from build123d import *

# Parameters (mm, degrees)
F1_DEPTH = 12
F2_SIZE  = 10


with BuildPart() as f1:
    # F0 (on Front) → F1 (new body)
    with BuildSketch(Plane.XZ):
        with BuildLine():
            Line((1, -45), (45, -45))
            Line((45, -45), (45, 45))
            Line((45, 45), (1, 45))
            Line((1, 45), (1, 24.096539))
            ThreePointArc((1, 24.096539), (0, 23.096539), (-1, 24.096539))
            Line((-1, 24.096539), (-1, 45))
            Line((-1, 45), (-45, 45))
            Line((-45, 45), (-45, -45))
            Line((-45, -45), (-1, -45))
            Line((-1, -45), (-1, -24.096539))
            ThreePointArc((-1, -24.096539), (0, -23.096539), (1, -24.096539))
            Line((1, -24.096539), (1, -45))
        make_face()
        with BuildLine():
            ThreePointArc((-6.732051, -7.660254), (-4, -6.928203), (-3.267949, -9.660254))
            Line((-3.267949, -9.660254), (-15.767949, -31.310889))
            ThreePointArc((-15.767949, -31.310889), (-18.5, -32.04294), (-19.232051, -29.310889))
            Line((-19.232051, -29.310889), (-6.732051, -7.660254))
        make_face(mode=Mode.SUBTRACT)
        with BuildLine():
            ThreePointArc((3.267949, -9.660254), (4, -6.928203), (6.732051, -7.660254))
            Line((6.732051, -7.660254), (19.232051, -29.310889))
            ThreePointArc((19.232051, -29.310889), (18.5, -32.04294), (15.767949, -31.310889))
            Line((15.767949, -31.310889), (3.267949, -9.660254))
        make_face(mode=Mode.SUBTRACT)
        with BuildLine():
            Line((-35, 2), (-10, 2))
            ThreePointArc((-10, 2), (-8, 0), (-10, -2))
            Line((-10, -2), (-35, -2))
            ThreePointArc((-35, -2), (-37, 0), (-35, 2))
        make_face(mode=Mode.SUBTRACT)
        with BuildLine():
            ThreePointArc((-3.267949, 9.660254), (-4, 6.928203), (-6.732051, 7.660254))
            Line((-6.732051, 7.660254), (-19.232051, 29.310889))
            ThreePointArc((-19.232051, 29.310889), (-18.5, 32.04294), (-15.767949, 31.310889))
            Line((-15.767949, 31.310889), (-3.267949, 9.660254))
        make_face(mode=Mode.SUBTRACT)
        with BuildLine():
            ThreePointArc((6.732051, 7.660254), (4, 6.928203), (3.267949, 9.660254))
            Line((3.267949, 9.660254), (15.767949, 31.310889))
            ThreePointArc((15.767949, 31.310889), (18.5, 32.04294), (19.232051, 29.310889))
            Line((19.232051, 29.310889), (6.732051, 7.660254))
        make_face(mode=Mode.SUBTRACT)
        with BuildLine():
            ThreePointArc((10, -2), (8, 0), (10, 2))
            Line((10, 2), (35, 2))
            ThreePointArc((35, 2), (37, 0), (35, -2))
            Line((35, -2), (10, -2))
        make_face(mode=Mode.SUBTRACT)
    extrude(amount=F1_DEPTH)

    # F2
    f2_edges = [f1.edges().sort_by_distance(p)[0] for p in [
        (45, -6, 45),
        (45, -6, -45),
        (-45, -6, 45),
        (-45, -6, -45),
    ]]
    chamfer(f2_edges, length=F2_SIZE)


solid = f1.part
Work out the finished part from the listing and answer in its coordinate system (mm). A direction names the side the tool comes from. Coordinates: 2 decimals unless noted, no trailing zeros. Write each loop counter-clockwise with the first axis right and the second up, starting at its lowest first coordinate (ties: lowest second). Pieces come first, ordered by that corner, then holes. Notation, with made-up numbers: M 35,68.25 L 60,68.25 A36 ccw 60,102.25 Z; hole C 13.5,86.5 d4. An arc over 180 degrees is marked long. Use one line per item in the form item = value. Start each with the question number.
1. A tool of negligible diameter and unlimited length cuts with its end or side. For faces 1 (the face through (-1, -6, -35)), 2 (the face through (40, -6, 40)), 3 (the face through (-37, -6, 0)), from which of +Z, -Z, +X, -X, +Y, -Y can it reach the whole face along a straight path? Write none if from no direction.
2. The mould has two halves that part along Z. Classify faces 4 (the face through (18, -6, -45)), 5 (the face through (9.605, -5.916, -20.637)), 6 (the face through (-1, -6, 34)), 7 (the face through (0.022, -5.916, 23.097)): released by +Z, released by -Z, zero draft, split by the parting line, or undercut.
3. The part is cut by section A-A (x = 17.5). Give the vertices of the cut face in (y, z), plus the area to 3 significant figures.
4. The part is cut by section B-B (z = 0). Give the vertices of the cut face in (x, y), plus the area to 3 significant figures.
5. The part is cut by section D-D (z = 28). Give the vertices of the cut face in (x, y).
6. The part is cut by section C-C (x = -32). Give the vertices of the cut face in (y, z), plus the area to 3 significant figures.
7. This flat-tipped pin is pushed along its axis until it touches: P1, Ø3, axis at x = 6, z = 9, coming from the +Y side. Where does it stop, or does it pass through?
8. Straight lines are drawn through the part: probe 1 along Z at (x, y) = (24.5, -7.75); probe 2 along X at (y, z) = (-10, -29.5); probe 3 along X at (y, z) = (-8.5, 9.5). For each, find the intervals that lie inside material, in ascending order. Write a range as from..to.
Evaluation:
q1.face_1 = -Z, +Y, -Y
q1.face_2 = +Z, +X, +Y, -Y
q1.face_3 = +Y, -Y
q2.face_4 = released by -Z
q2.face_5 = undercut
q2.face_6 = zero draft
q2.face_7 = released by +Z
q3.outline = M -12,-45 L 0,-45 L 0,-32.31 L -12,-32.31 Z; M -12,-26.31 L 0,-26.31 L 0,-2 L -12,-2 Z; M -12,2 L 0,2 L 0,26.31 L -12,26.31 Z; M -12,32.31 L 0,32.31 L 0,45 L -12,45 Z
q3.area = 888 mm^2
q4.outline = M -45,-12 L -37,-12 L -37,0 L -45,0 Z; M -8,-12 L 8,-12 L 8,0 L -8,0 Z; M 37,-12 L 45,-12 L 45,0 L 37,0 Z
q4.area = 384 mm^2
q5.outline = M -45,-12 L -18.48,-12 L -18.48,0 L -45,0 Z; M -13.86,-12 L -1,-12 L -1,0 L -13.86,0 Z; M 1,-12 L 13.86,-12 L 13.86,0 L 1,0 Z; M 18.48,-12 L 45,-12 L 45,0 L 18.48,0 Z
q6.outline = M -12,-45 L 0,-45 L 0,-2 L -12,-2 Z; M -12,2 L 0,2 L 0,45 L -12,45 Z
q6.area = 1,030 mm^2
q7.P1 = 0
q8.probe_1 = -45..-2, 2..45
q8.probe_2 = -45..-19.33, -14.72..-1, 1..14.72, 19.33..45
q8.probe_3 = -45..-7.79, -3.18..3.18, 7.79..45
